The drawing under review shows one solid part. Ordinate dimensions are in mm from its lowest x, y, z. A direction names the side the tool comes from. Coordinates: 2 decimals unless noted, no trailing zeros. Order: outer loops, then holes, each group sorted by start corner. A loop starts at its lowest first (then second) coordinate and runs counter-clockwise, first axis right, second up.
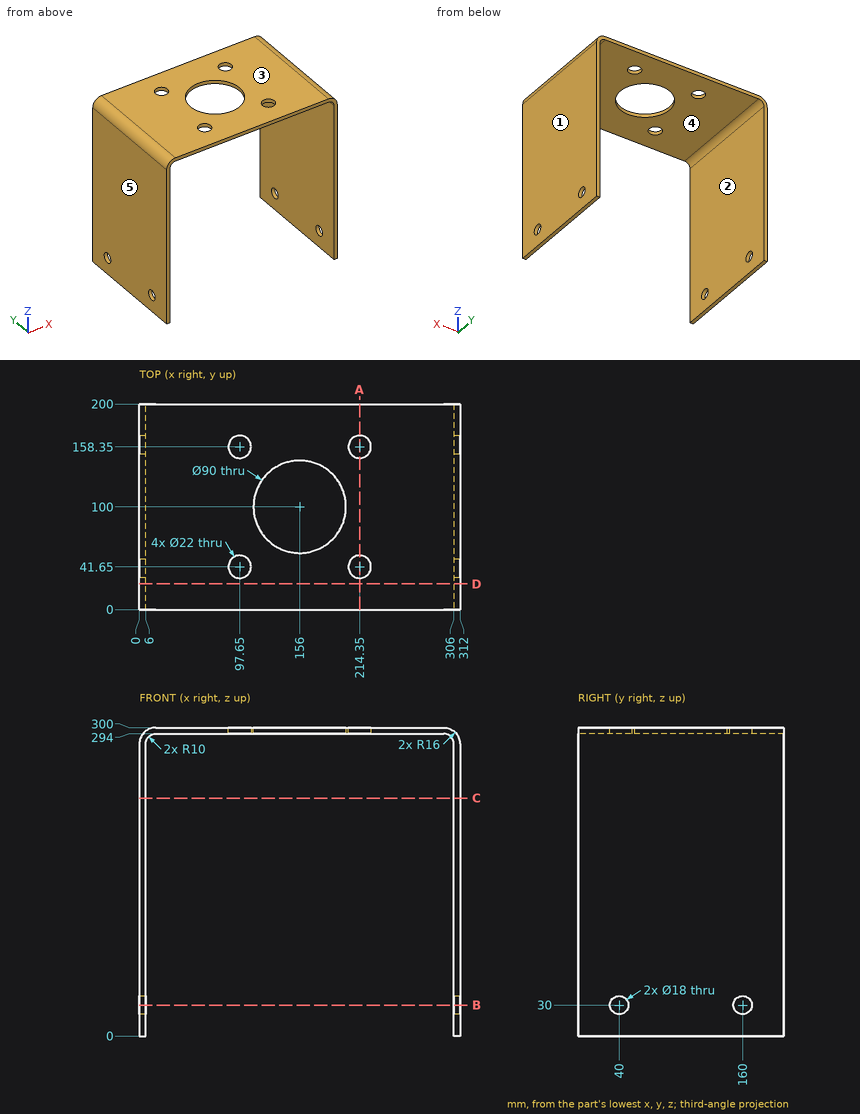
1. Take a section at C-C, the plane z = 231.5. Give the boundary of the cut face in (x, y).
Answer below:
outline: (0, 0) - (6, 0) - (6, 200) - (0, 200) - close; (306, 0) - (312, 0) - (312, 200) - (306, 200) - close
2. Take a section at B-B, the plane z = 30. Give the boundary of the cut face in (x, y).
Answer below:
outline: (0, 0) - (6, 0) - (6, 31) - (0, 31) - close; (0, 49) - (6, 49) - (6, 151) - (0, 151) - close; (0, 169) - (6, 169) - (6, 200) - (0, 200) - close; (306, 0) - (312, 0) - (312, 31) - (306, 31) - close; (306, 49) - (312, 49) - (312, 151) - (306, 151) - close; (306, 169) - (312, 169) - (312, 200) - (306, 200) - close
3. The part is to be moulded in two halves that separate along X. For the marked faces 3, 4 and 5, say which applies: +X half, -X half, draft (parallel to the pull), parting line (faces both ways), or undercut.
Answer below:
face 3: draft
face 4: undercut
face 5: -X half
4. Clearance check with flat-ended pins moving along their axes: pin 1 Ø6 at (x, y) = (62.5, 137) entering from -Z; pin 2 Ø11 at (y, z) = (40, 30) entering from -X. State where each tip first meets the part, or that it passes through.
Answer below:
pin 1: stops at z = 294
pin 2: passes through
5. Take a section at D-D, the plane y = 25. Give the boundary of the cut face in (x, z), plus the area to 3 significant figures.
Answer below:
outline: (0, 0) - (6, 0) - (6, 284) arc R10 cw to (16, 294) - (296, 294) arc R10 cw to (306, 284) - (306, 0) - (312, 0) - (312, 284) arc R16 ccw to (296, 300) - (16, 300) arc R16 ccw to (0, 284) - close
area: 5,330 mm2
6. To check wall thickness, follow L1, parallel to Y at x = 3.9, z = 30; L2, parallel to Y at x = 97, z = 295; L3, parallel to X at y = 106, z = 230. State the ranges of each line that lie inside material, in increasing order.
Answer below:
L1: y = 0 to 31, 49 to 151, 169 to 200
L2: y = 0 to 30.67, 52.63 to 147.37, 169.33 to 200
L3: x = 0 to 6, 306 to 312
7. Machinability: for the marked faces 1 and 2, which of the approach directions +Z, -Z, +X, -X, +Y, -Y give a long, thin tool a straight path to every point of the face, cutting with its end or side? Answer none if there is none.
Answer below:
face 1: +Z, -Z, +X, +Y, -Y
face 2: -Z, +Y, -Y
8. Take a section at A-A, the plane x = 214.35. Give the boundary of the cut face in (y, z), plus the area to 3 significant figures.
Answer below:
outline: (0, 294) - (30.65, 294) - (30.65, 300) - (0, 300) - close; (52.65, 294) - (147.35, 294) - (147.35, 300) - (52.65, 300) - close; (169.35, 294) - (200, 294) - (200, 300) - (169.35, 300) - close
area: 936 mm2
